Could you check a few things on this model? Use its own coordinates, in mm. Face numbers are marked on the shaded views. A direction names the side the tool comes from. Round coordinates to 2 decimals unless told otherwise and drop trailing zeros. Loops run counter-clockwise (first coordinate to the right, second up) from the corner with the lowest first, then second, coordinate; pieces in that order, holes last. Notation, with made-up numbers: (6.25, 38.5) -> (20.25, 38.5) arc R32 ccw to (20.25, 69.5) -> close; hole circle Ø7 at (30.25, -31.5). An arc over 180 degrees is marked (long way). Put each result on its own line as item: value. Start each with the question number.
1. Which directions (+Z, -Z, +X, -X, +Y, -Y) give clear straight access to the entire face, cutting with the end or side of a thin tool? Please do the marked faces 1 and 2.
2. Imagine slicing it at C-C, the plane z = -1.7. Please give me the cut outline in (x, y).
3. I need wall thicknesses on line 1 (Y direction, x = 0.15, z = 2.1); line 2 (Y direction, x = -1, z = 1.3); line 3 (X direction, y = 0.5, z = -1.2). Which ranges of each line are inside material? Lowest first, please. Write a range as [from, to].
4. I'm going to push flat-ended pins straight in: P1, Ø3, axis at y = 7.5, z = -1.5, coming from the -X side; P2, Ø1, axis at x = 0, z = -0.5, coming from the +Y side; P3, Ø3, axis at y = 3, z = 2, coming from the -X side. Where does each tip first touch, or does it pass through?
5. Imagine slicing it at D-D, the plane x = 2.15. Please give me the cut outline in (y, z), and give its area (3 significant figures).
6. If we mould it in two halves opening along Z, with no side actions, what happens to the marked faces 3, 4 and 5? For each: pulls with the +Z half, pulls with the -Z half, needs draft (parallel to the pull), parting line crosses it, or undercut.
7. Imagine slicing it at B-B, the plane y = 1. Please give me the cut outline in (x, z) (3 decimals).
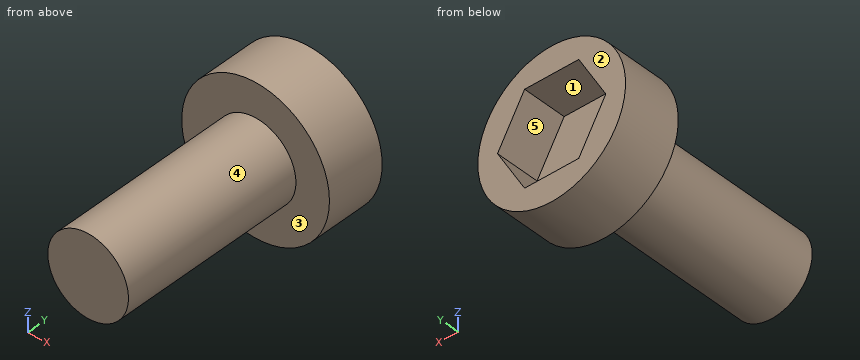
Autodesk Inventor part; units mm, degrees
ref_plane "YZ Plane" through (0, 0, 0) normal (1, 0, 0) x (0, 1, 0)
ref_plane "XZ Plane" through (0, 0, 0) normal (0, 1, 0) x (-1, 0, 0)
ref_plane "XY Plane" through (0, 0, 0) normal (0, 0, 1) x (1, 0, 0)
sketch "Sketch1" plane through (0, 0, 0) normal (0, 1, 0) x (-1, 0, 0)
  circle A0 centre (0, 0) radius 1.365
  dimension "d0" = 2.73
extrude "Extrusion1" add sketch "Sketch1" along normal blind 6.35
sketch "Sketch2" plane through (0, 6.35, 0) normal (0, 1, 0) x (1, 0, 0)
  circle A0 centre (0, 0) radius 2.5
  dimension "d3" = 5
extrude "Extrusion2" add sketch "Sketch2" along normal blind 2
sketch "Sketch3" plane through (0, 8.35, 0) normal (0, 1, 0) x (1, 0, 0)
  circle A0 centre (0, 0) radius 1.365
  line L0 (-1.8331, 0) -> (-0.9165, 1.5875)
  line L1 (-0.9165, 1.5875) -> (0.9165, 1.5875)
  line L2 (0.9165, 1.5875) -> (1.8331, 0)
  line L3 (1.8331, 0) -> (0.9165, -1.5875)
  line L4 (0.9165, -1.5875) -> (-0.9165, -1.5875)
  line L5 (-0.9165, -1.5875) -> (-1.8331, 0)
  dimension "d6" = 3.175
extrude "Extrusion3" cut sketch "Sketch3" against normal blind 1.5 contours A0 | L0 L1 L2 L3 L4 L5
thread "Thread1"
properties part number "Electronics Mounting bolt" material "Steel, Galvanized"
Entries:
1. face 1: +Y
1. face 2: +Z, -Z, +X, -X, +Y
2. outline: (-1.83, 6.35) -> (1.83, 6.35) -> (1.83, 8.35) -> (-1.83, 8.35) -> close
3. line 1: [6.35, 8.35]
3. line 2: [6.35, 6.85]
3. line 3: [-0.65, 0.65]
4. P1: x = -2.5
4. P2: y = 6.85
4. P3: x = -1.27
5. outline: (6.35, -1.28) -> (8.35, -1.28) -> (8.35, 1.28) -> (6.35, 1.28) -> close
5. area: 5.10 mm^2
6. face 3: needs draft
6. face 4: parting line crosses it
6. face 5: undercut
7. outline: circle Ø2.73 at (0, 0)
